from build123d import *

# Parameters (mm, degrees)
SKETCH1_R               = 30
SKETCH1_R_2             = 1
BOSS_EXTRUDE1_DEPTH     = 2
CUT_EXTRUDE1_DEPTH      = 43.473521163
CUT_EXTRUDE1_DEPTH_BACK = 43.473521163


with BuildPart() as part:
    # Sketch1 → Boss-Extrude1 (new body)
    with BuildSketch(Plane(origin=(0, 0, 0), x_dir=(1, 0, 0), z_dir=(0, 1, 0))):
        with Locations(Location((0, 0, 0), (0, 0, 270))):
            Circle(SKETCH1_R)
        with Locations(Location((-11.874342087, 22, 0), (0, 0, 270))):
            Circle(SKETCH1_R_2, mode=Mode.SUBTRACT)
        with Locations(Location((11.874342087, 22, 0), (0, 0, 270))):
            Circle(SKETCH1_R_2, mode=Mode.SUBTRACT)
        with Locations(Location((11.874342087, -22, 0), (0, 0, 270))):
            Circle(SKETCH1_R_2, mode=Mode.SUBTRACT)
        with Locations(Location((-11.874342087, -22, 0), (0, 0, 270))):
            Circle(SKETCH1_R_2, mode=Mode.SUBTRACT)
        with Locations(Location((-11.874342087, 16.093476939, 0), (0, 0, 270))):
            Circle(SKETCH1_R_2, mode=Mode.SUBTRACT)
        with Locations(Location((11.874342087, 16.093476939, 0), (0, 0, 270))):
            Circle(SKETCH1_R_2, mode=Mode.SUBTRACT)
        with Locations(Location((11.874342087, -16.093476939, 0), (0, 0, 270))):
            Circle(SKETCH1_R_2, mode=Mode.SUBTRACT)
        with Locations(Location((-11.874342087, -16.093476939, 0), (0, 0, 270))):
            Circle(SKETCH1_R_2, mode=Mode.SUBTRACT)
        with Locations(Location((-15.612494996, 12.5, 0), (0, 0, 270))):
            Circle(SKETCH1_R_2, mode=Mode.SUBTRACT)
        with Locations(Location((15.612494996, 12.5, 0), (0, 0, 270))):
            Circle(SKETCH1_R_2, mode=Mode.SUBTRACT)
        with Locations(Location((15.612494996, -12.5, 0), (0, 0, 270))):
            Circle(SKETCH1_R_2, mode=Mode.SUBTRACT)
        with Locations(Location((-15.612494996, -12.5, 0), (0, 0, 270))):
            Circle(SKETCH1_R_2, mode=Mode.SUBTRACT)
    extrude(amount=BOSS_EXTRUDE1_DEPTH)

    # Sketch2 → Cut-Extrude1 (cut, two sides: drawn at the far end of the back side and taken through both)
    with BuildSketch(Plane(origin=(0, 2, 0), x_dir=(1, 0, 0), z_dir=(0, 1, 0)).offset(-CUT_EXTRUDE1_DEPTH_BACK)):
        with BuildLine():
            Line((-5, 8), (-0.5, 8))
            Line((-0.5, 8), (-0.5, 10.25))
            Line((-0.5, 10.25), (0.5, 10.25))
            Line((0.5, 10.25), (0.5, 8))
            Line((0.5, 8), (5, 8))
            ThreePointArc((5, 8), (5.707106781, 7.707106781), (6, 7))
            Line((6, 7), (6, -16))
            ThreePointArc((6, -16), (5.707106781, -16.707106781), (5, -17))
            Line((5, -17), (0.5, -17))
            Line((0.5, -17), (0.5, -19.25))
            Line((0.5, -19.25), (-0.5, -19.25))
            Line((-0.5, -19.25), (-0.5, -17))
            Line((-0.5, -17), (-5, -17))
            ThreePointArc((-5, -17), (-5.707106781, -16.707106781), (-6, -16))
            Line((-6, -16), (-6, 7))
            ThreePointArc((-6, 7), (-5.707106781, 7.707106781), (-5, 8))
        make_face()
    extrude(amount=CUT_EXTRUDE1_DEPTH + CUT_EXTRUDE1_DEPTH_BACK, mode=Mode.SUBTRACT)


solid = part.part
The model under review builds one solid part; all positions refer to its coordinate system, in mm. A direction names the side the tool comes from. Round coordinates to 2 decimals unless told otherwise and drop trailing zeros. Write each loop counter-clockwise with the first axis right and the second up, starting at its lowest first coordinate (ties: lowest second). Pieces come first, ordered by that corner, then holes. Notation, with made-up numbers: (-34, -9.75) - (-29, -9.75) arc R21 cw to (-29, 25.25) - close; hole circle Ø7 at (3.25, 37). An arc over 180 degrees is marked (long way). One line per item, written item: value. Start each with the question number.
1. Consider section C-C on z = -22. Write out the cut boundary in (x, y), and give its area (3 significant figures).
2. Clearance check with flat-ended pins moving along their axes: P1, Ø0.6, axis at y = 0.5, z = 17.5, coming from the -X side; P2, Ø1, axis at y = 1, z = -0.5, coming from the -X side; P3, Ø2.5, axis at x = 11.87, z = 22, coming from the -Y side; P4, Ø1, axis at x = 15, y = 1.5, coming from the -Z side. State where each tip first meets the part, or that it passes through.
3. Consider section A-A on z = 0. Write out the cut boundary in (x, y), and give its area (3 significant figures).
4. The part is to be moulded in two halves that separate along X. For faces 1 (the face through (-6.2, 0, -0.4)), 2 (the face through (1.32, 0.99, -29.97)), 3 (the face through (11.9, 1, -23)), say which applies: released by +X, released by -X, zero draft, split by the parting line, or undercut.
5. Consider section B-B on y = 1.55. State how many separate pieces and enclosed holes the cut face has, and give its area (3 significant figures).
6. Machinability: for faces 4 (the face through (-6.2, 2, -0.4)), 5 (the face through (-3, 1, 17)), which of the approach directions +Z, -Z, +X, -X, +Y, -Y give a long, thin tool a straight path to every point of the face, cutting with its end or side? Answer none if there is none.
7. To check wall thickness, follow L1, parallel to X at y = 0.2, z = -22; L2, parallel to X at y = 1.1, z = 12.5; L3, parallel to Z at x = 1, y = 1.45. State the ranges of each line that lie inside material, in increasing order. Write a range as from..to.
8. Consider section D-D on x = 2. Write out the cut boundary in (y, z).
Checks:
1. outline: (-20.4, 0) - (-12.87, 0) - (-12.87, 2) - (-20.4, 2) - close; (-10.87, 0) - (10.87, 0) - (10.87, 2) - (-10.87, 2) - close; (12.87, 0) - (20.4, 0) - (20.4, 2) - (12.87, 2) - close
1. area: 73.6 mm^2
2. P1: stops at x = -24.58
2. P2: stops at x = -30
2. P3: stops at y = 0
2. P4: stops at z = -26.26
3. outline: (-30, 0) - (-6, 0) - (-6, 2) - (-30, 2) - close; (6, 0) - (30, 0) - (30, 2) - (6, 2) - close
3. area: 96.0 mm^2
4. face 1: zero draft
4. face 2: split by the parting line
4. face 3: undercut
5. separate pieces: 1
5. enclosed holes: 13
5. area: 2,490 mm^2
6. face 4: +Z, -Z, +X, -X, +Y
6. face 5: +Y, -Y
7. L1: x = -20.4..-12.87, -10.87..10.87, 12.87..20.4
7. L2: x = -27.27..-16.61, -14.61..-6, 6..14.61, 16.61..27.27
7. L3: z = -29.98..-8, 17..29.98
8. outline: (0, -29.93) - (2, -29.93) - (2, -8) - (0, -8) - close; (0, 17) - (2, 17) - (2, 29.93) - (0, 29.93) - close
